Autodesk Inventor part; units mm, degrees
ref_plane "YZ Plane" through (0, 0, 0) normal (1, 0, 0) x (0, 1, 0)
ref_plane "XZ Plane" through (0, 0, 0) normal (0, 1, 0) x (-1, 0, 0)
ref_plane "XY Plane" through (0, 0, 0) normal (0, 0, 1) x (1, 0, 0)
sketch "Sketch1" plane through (0, 0, 0) normal (0, 1, 0) x (-1, 0, 0)
  line L0 (0, 0) -> (-42.4, 0)
  line L1 (-42.4, -20) -> (-42.4, -51.2)
  line L2 (-42.4, -51.2) -> (0, -51.2)
  line L3 (0, -51.2) -> (0, -20)
  line L4 (-21.2, 0) -> (-6.45, 0)
  line L5 (-6.45, 0) -> (-28.15, 0)
  line L6 (-21.2, 0) -> (0.55, 0)
  line L7 (0.55, 0) -> (-30.65, 0)
  line L8 (-21.2, 0) -> (-5.6, 0)
  line L9 (-5.6, 0) -> (-36.8, 0)
  arc A0 (-35.2, -8.4) -> (-38.4, -8.4) centre (-36.8, -8.4) ccw
  arc A1 (-38.4, -46.5) -> (-35.2, -46.5) centre (-36.8, -46.5) ccw
  arc A2 (-4, -8.4) -> (-7.2, -8.4) centre (-5.6, -8.4) ccw
  arc A3 (-7.2, -46.5) -> (-4, -46.5) centre (-5.6, -46.5) ccw
  line L10 (0, 0) -> (0, -20)
  line L11 (0, -20) -> (20, -20)
  line L12 (20, -20) -> (20, 0)
  line L13 (20, 0) -> (0, 0)
  line L14 (-42.4, -20) -> (-62.4, -20)
  line L15 (-62.4, -20) -> (-62.4, 0)
  line L16 (-62.4, 0) -> (-42.4, 0)
  line L17 (-4, -46.5) -> (-4, -8.4)
  line L18 (-7.2, -8.4) -> (-7.2, -46.5)
  line L19 (-35.2, -46.5) -> (-35.2, -8.4)
  line L20 (-38.4, -8.4) -> (-38.4, -46.5)
  dimension "d0" = 42.4
  dimension "d1" = 51.2
  dimension "d41" = 15.6
  dimension "d42" = 31.2
  dimension "d50" = 3.2
  dimension "d56" = 3.2
  dimension "d57" = 3.2
  dimension "d63" = 3.2
  dimension "d67" = 8.4
  dimension "d77" = 8.4
  dimension "d81" = 20
  dimension "d82" = 20
  dimension "d83" = 20
extrude "Extrusion3" add sketch "Sketch1" along normal blind 2
fillet "Fillet2" radius 3.175 2 edges at (0, 1, -51.2) (42.4, 1, -51.2)
sketch "Sketch2" plane through (0, 2, 0) normal (0, 1, 0) x (1, 0, 0)
  circle A0 centre (-10, 10) radius 2.125
  line L0 (-20, 0) -> (62.4, 0)
  line L1 (38.17, 0) -> (48.17, 0)
  line L2 (62.4, 0) -> (52.4, 0)
  line L3 (-20, 0) -> (62.4, 0)
  line L4 (52.4, 0) -> (52.4, 10)
  circle A1 centre (52.4, 10) radius 2.125
  point P0 (0, 0)
  dimension "d85" = 4.25
  dimension "d92" = 10
  dimension "d93" = 10
  dimension "d94" = 4.25
extrude "Extrusion4" cut sketch "Sketch2" against normal blind 2
fillet "Fillet3" radius 5 4 edges at (62.4, 1, -20) (62.4, 1, 0) (-20, 1, 0) (-20, 1, -20)
properties part number "Motor Attachment Small 3.0"
Here's how the part is built. I have some questions about the finished solid (model axes, mm). A direction names the side the tool comes from. Round coordinates to 2 decimals unless told otherwise and drop trailing zeros. Order: outer loops, then holes, each group sorted by start corner. A loop starts at its lowest first (then second) coordinate and runs counter-clockwise, first axis right, second up. Notation, with made-up numbers: M 13.25,87.25 L 39.25,87.25 A26 cw 39.25,114.25 Z; hole C -9,-8 d8. An arc over 180 degrees is marked long. Return JSON: item names as keys, results as strings. Group by question number.
1. If we section it at A-A on x = 52.4: List the corners of the cut face in (y, z) for me (3 decimals), then the cut area to 3 significant figures.
2. If we mould it in two halves opening along Z, with no side actions, what happens to faces 4 (the face through (-7, 1, -20)), 5 (the face through (-10.461, 1.014, -7.926)), 6 (the face through (0, 1, -34)), 7 (the face through (7.2, 1, -27))? For each: pulls with the +Z half, pulls with the -Z half, needs draft (parallel to the pull), parting line crosses it, or undercut.
3. On a 3-axis mill with a long thin cutter (end or side, diameter ignored), from which of +Z, -Z, +X, -X, +Y, -Y can I reach the whole of each face in a straight line? I mean faces 1 (the face through (38.4, 1, -27)), 2 (the face through (60.9, 1.01, -1.43)), 3 (the face through (50, 1, -20)). Say none if no direction works.
4. I'm going to push flat-ended pins straight in: pin 1 Ø5 at (x, z) = (-10, -10) entering from -Y; pin 2 Ø0.6 at (y, z) = (1, -34) entering from -X; pin 3 Ø0.6 at (y, z) = (0.5, -29) entering from +X. Where does each tip first touch, or does it pass through?
5. If we section it at D-D on z = -29: List the corners of the cut face in (x, y) for me.
6. Please list where these lines run through material, in increasing order: probe 1 along X at (y, z) = (1.1, -33); probe 2 along X at (y, z) = (1.45, -10) (3 decimals); probe 3 along Z at (x, y) = (-10, 1.35) (3 decimals).
7. If we section it at B-B on z = -13: List the corners of the cut face in (x, y) for me, then the cut area to 3 significant figures.
8. If we section it at C-C on y = 1.5: List the corners of the cut face in (x, z) for me (3 decimals), then the cut area to 3 significant figures.
Reply:
{
 "1": {"outline": "M 0,-20 L 2,-20 L 2,-12.125 L 0,-12.125 Z; M 0,-7.875 L 2,-7.875 L 2,0 L 0,0 Z", "area": "31.5 mm^2"},
 "2": {"face 4": "pulls with the -Z half", "face 5": "undercut", "face 6": "needs draft", "face 7": "undercut"},
 "3": {"face 1": "+Y, -Y", "face 2": "+Z, +X, +Y, -Y", "face 3": "-Z, +X, +Y, -Y"},
 "4": {"pin 1": "y = 0", "pin 2": "x = 0", "pin 3": "x = 42.4"},
 "5": {"outline": "M 0,0 L 4,0 L 4,2 L 0,2 Z; M 7.2,0 L 35.2,0 L 35.2,2 L 7.2,2 Z; M 38.4,0 L 42.4,0 L 42.4,2 L 38.4,2 Z"},
 "6": {"probe 1": "0 to 4, 7.2 to 35.2, 38.4 to 42.4", "probe 2": "-20 to -12.125, -7.875 to 4, 7.2 to 35.2, 38.4 to 50.275, 54.525 to 62.4", "probe 3": "-20 to -12.125, -7.875 to 0"},
 "7": {"outline": "M -20,0 L 4,0 L 4,2 L -20,2 Z; M 7.2,0 L 35.2,0 L 35.2,2 L 7.2,2 Z; M 38.4,0 L 62.4,0 L 62.4,2 L 38.4,2 Z", "area": "152 mm^2"},
 "8": {"outline": "M -20,-15 A5 ccw -15,-20 L 0,-20 L 0,-48.025 A3.175 ccw 3.175,-51.2 L 39.225,-51.2 A3.175 ccw 42.4,-48.025 L 42.4,-20 L 57.4,-20 A5 ccw 62.4,-15 L 62.4,-5 A5 ccw 57.4,0 L -15,0 A5 ccw -20,-5 Z; hole C -10,-10 d4.25; hole M 4,-46.5 A1.6 ccw 7.2,-46.5 L 7.2,-8.4 A1.6 ccw 4,-8.4 Z; hole M 35.2,-46.5 A1.6 ccw 38.4,-46.5 L 38.4,-8.4 A1.6 ccw 35.2,-8.4 Z; hole C 52.4,-10 d4.25", "area": "2,660 mm^2"}
}
